Autodesk Fusion 360 part; units mm, degrees
sketch "Sketch1" plane through (0, 0, 0) normal (0, 1, 0) x (1, 0, 0)
  line L0 (0, 0) -> (124, 0)
  line L1 (124, 0) -> (124, 40)
  line L2 (124, 40) -> (0, 40)
  line L3 (0, 40) -> (0, 0)
  circle A0 centre (14, 20) radius 5
  circle A1 centre (110, 20) radius 5
  line L4 (0, 20) -> (3, 0)
  line L5 (0, 20) -> (3, 40)
  line L6 (124, 20) -> (121, 0)
  line L7 (124, 20) -> (121, 40)
  circle A2 centre (62, 20) radius 20
  circle A3 centre (62, 20) radius 10
  line L8 (62, 33) -> (90, 33)
  line L9 (90, 33) -> (90, 7)
  line L10 (90, 7) -> (62, 7)
  line L11 (62, 7) -> (62, 33)
  dimension "d1" = 124
  dimension "d2" = 40
  dimension "d3" = 14
  dimension "d4" = 14
  dimension "d5" = 3
  dimension "d6" = 3
  dimension "d7" = 3
  dimension "d8" = 3
  dimension "d9" = 40
  dimension "d10" = 62
  dimension "d11" = 20
  dimension "d12" = 28
  dimension "d13" = 26
  dimension "d14" = 13
  dimension "d15" = 28
extrude "Extrude1" add sketch "Sketch1" along normal blind 16 contours L0 L2 L4 L5 A2 | L0 L2 L6 L7 A2 L8 L9 L10
extrude "Extrude2" add sketch "Sketch1" along normal blind 46 contours A2 A3 L8 L10 L11 | A2 A3 L8 L10 L11 | A2 L8 L9 L10
extrude "Extrude3" add sketch "Sketch1" against normal blind 14 contours A2 A3 L8 L10 L11 | A2 A3 L8 L10 L11
equation "d10 = ( 124 / 2 ) * 1 mm"
Read the model definition and answer for the solid it produces. Units are mm, in the model's axes. A direction names the side the tool comes from. Coordinates: 2 decimals unless noted, no trailing zeros. Loops run counter-clockwise (first coordinate to the right, second up) from the corner with the lowest first, then second, coordinate; pieces in that order, holes last.
Q1. Which of the six approach directions +Z, -Z, +X, -X, +Y, -Y give full straight-line access (tool end or side, diameter ignored) to faces 1 (the face through (84, 31, -33)), 2 (the face through (80.475, -6.902, -12.34)), 3 (the face through (84, 31, -7))?
Q2. The part is cut by section A-A on x = 11. Write down the section's boundary in (y, z).
Q3. Each of these flat-tipped pins is pushed along its axis until it touches: pin 1 Ø10 at (y, z) = (31, -11) entering from +X; pin 2 Ø1 at (x, z) = (14, -7) entering from -Y; pin 3 Ø5 at (x, z) = (94.5, -7.5) entering from +Y; pin 4 Ø8 at (x, y) = (48, 2) entering from +Z. Where does it stop, or does it pass through?
Q4. Consider probe 1 along X at (y, z) = (4, -20); probe 2 along Z at (x, y) = (62, 20); probe 3 along Z at (x, y) = (110, 8). Determine where each line is inside the solid, lowest interval first.
Q5. The part is cut by section D-D on y = -2.5. Write down the section's boundary in (x, z), and give its area (3 significant figures).
Q6. The mould has two halves that part along X. Classify faces 4 (the face through (114.619, 7.888, -21.915)), 5 (the face through (1.48, 7.89, -29.86)), 6 (the face through (52, 16, -20)), 7 (the face through (90, 31, -20)): +X half, -X half, draft (parallel to the pull), parting line (faces both ways), or undercut.
Q7. The part is cut by section C-C on x = 46. Write down the section's boundary in (y, z), and give its area (3 significant figures).
Q8. The part is cut by section B-B on y = 14. Write down the section's boundary in (x, z), and give its area (3 significant figures).
Results below:
1. face 1: -Z, +X, +Y
1. face 2: -Y
1. face 3: +Z, +X, +Y
2. outline: (0, -40) - (16, -40) - (16, -24) - (0, -24) - close; (0, -16) - (16, -16) - (16, 0) - (0, 0) - close
3. pin 1: stops at x = 90
3. pin 2: stops at y = 0
3. pin 3: stops at y = 16
3. pin 4: stops at z = 0
4. probe 1: x = 0 to 9, 19 to 52, 72 to 105, 115 to 124
4. probe 2: z = -40 to -30, -10 to 0
4. probe 3: z = -40 to -25, -15 to 0
5. outline: circle Ø40 at (62, -20); hole circle Ø20 at (62, -20)
5. area: 942 mm2
6. face 4: undercut
6. face 5: -X half
6. face 6: undercut
6. face 7: +X half
7. outline: (-14, -32) - (0, -32) - (0, -40) - (16, -40) - (16, -32) - (46, -32) - (46, -8) - (16, -8) - (16, 0) - (0, 0) - (0, -8) - (-14, -8) - close
7. area: 1,700 mm2
8. outline: (0, -20) - (3, -40) - (121, -40) - (124, -20) - (121, 0) - (3, 0) - close; hole circle Ø10 at (14, -20); hole circle Ø20 at (62, -20); hole circle Ø10 at (110, -20)
8. area: 4,370 mm2
